from build123d import *

# Parameters (mm, degrees)
F0_W     = 125.685974
F0_H     = 54.542944
F1_DEPTH = 25.4
F2_SIZE  = 12.7
F3_R     = 12.7


with BuildPart() as f1:
    # F0 (on Top) → F1 (new body)
    with BuildSketch(Plane.XY):
        Rectangle(F0_W, F0_H)
    extrude(amount=F1_DEPTH)

    # F2
    f2_edges = [f1.edges().sort_by_distance(p)[0] for p in [
        (0, -27.271472, 25.4),
    ]]
    chamfer(f2_edges, length=F2_SIZE)

    # F3
    f3_edges = [f1.edges().sort_by_distance(p)[0] for p in [
        (0, 27.271472, 25.4),
    ]]
    fillet(f3_edges, radius=F3_R)


solid = f1.part
Model file for the job. Use its own axes, mm. Round coordinates to 2 decimals unless told otherwise and drop trailing zeros. Order: outer loops, then holes, each group sorted by start corner. A loop starts at its lowest first (then second) coordinate and runs counter-clockwise, first axis right, second up.
(1) Pin check, flat tip, straight feed: pin 1 (1 mm diameter, centred on x = -26, z = 19, fed in from +Y). Stop position of the tip, or through.
(2) Band-saw the part on A-A (x = -25). List the corners of the cut face in (y, z), then the cut area to 3 significant figures.
(3) Band-saw the part on B-B (y = -16.5). List the corners of the cut face in (x, z), then the cut area to 3 significant figures.
(4) Band-saw the part on C-C (z = 22.5). List the corners of the cut face in (x, y), then the cut area to 3 significant figures.
(5) Drill centre lines: line 1 (Z direction, x = 15, y = -19); line 2 (Y direction, x = -53.5, z = 14.75); line 3 (Y direction, x = 45, z = 19.25). Where is each one in solid material? Low to high.
Verdict:
1. pin 1: stops at y = 25.87
2. outline: (-27.27, 0) - (27.27, 0) - (27.27, 12.7) arc R12.7 ccw to (14.57, 25.4) - (-14.57, 25.4) - (-27.27, 12.7) - close
2. area: 1,270 mm2
3. outline: (-62.84, 0) - (62.84, 0) - (62.84, 23.47) - (-62.84, 23.47) - close
3. area: 2,950 mm2
4. outline: (-62.84, -17.47) - (62.84, -17.47) - (62.84, 22.65) - (-62.84, 22.65) - close
4. area: 5,040 mm2
5. line 1: z = 0 to 20.97
5. line 2: y = -25.22 to 27.1
5. line 3: y = -20.72 to 25.45
